Work out the finished part from the listing and answer in its coordinate system (mm). A direction names the side the tool comes from. Coordinates: 2 decimals unless noted, no trailing zeros. Loops run counter-clockwise (first coordinate to the right, second up) from the corner with the lowest first, then second, coordinate; pieces in that order, holes last.
```python
from build123d import *

# Parameters (mm, degrees)
BOSS_EXTRUDE1_DEPTH             = 7.5
F_2_CLEARANCE_HOLE1_D           = 2.2606
F_3_CLEARANCE_HOLE1_D           = 2.6416
F_3_CLEARANCE_HOLE1_CSINK_D     = 4.318
F_3_CLEARANCE_HOLE1_CSINK_ANGLE = 90
FILLET1_R                       = 3


with BuildPart() as part:
    # Sketch3 → Boss-Extrude1 (new body, symmetric)
    with BuildSketch(Plane(origin=(0, 0, 0), x_dir=(1, 0, 0), z_dir=(0, 1, 0))):
        Polygon((0, 0), (0, 20), (3.175, 20), (3.175, 3.175), (15, 3.175), (15, 0), align=None)
    extrude(amount=BOSS_EXTRUDE1_DEPTH, both=True)

    # #2 Clearance Hole1 (through all)
    with Locations(Plane.XY):
        with Locations((10, -3.25), (10, 3.25)):
            Hole(F_2_CLEARANCE_HOLE1_D / 2)

    # #3 Clearance Hole1 (through all)
    with Locations(Plane(origin=(3.175, 0, 0), x_dir=(0, 0, -1), z_dir=(1, 0, 0))):
        with Locations((7.3375, 0), (15.8375, 0)):
            CounterSinkHole(F_3_CLEARANCE_HOLE1_D / 2, F_3_CLEARANCE_HOLE1_CSINK_D / 2, counter_sink_angle=F_3_CLEARANCE_HOLE1_CSINK_ANGLE)

    # Fillet1
    fillet1_edges = [part.edges().sort_by_distance(p)[0] for p in [
        (1.5875, 7.5, -20),
        (1.5875, -7.5, -20),
        (15, -7.5, -1.5875),
        (15, 7.5, -1.5875),
    ]]
    fillet(fillet1_edges, radius=FILLET1_R)


solid = part.part
```
1. A cutting plane is placed at C-C, the plane z = -1.25. Give the vertices of the cut face in (x, y), then the cut area to 3 significant figures.
2. For faces 4 (the flat face through (8, 0, 0)), 5 (the flat face through (9, 0, -3.175)), determine the directions among +Z, -Z, +X, -X, +Y, -Y from which every point of the face is accessible in a straight line to the end or side of a thin tool.
3. Determine the mould class of faces 1 (the cylindrical face through (11.13, -3.2, -1.61)), 2 (the cylindrical face through (1.15, -0.8, -8.39)), 3 (the cylindrical face through (1.61, 6.6, -19.14)) for opening direction Z: released by +Z, released by -Z, zero draft, split by the parting line, or undercut.
4. A cutting plane is placed at A-A, the plane y = 3.25. Give the vertices of the cut face in (x, z) (3 decimals), then the cut area to 3 significant figures.
5. Straight lines are drawn through the part: probe 1 along Z at (x, y) = (0.9, 0); probe 2 along Y at (x, z) = (10, -1.3); probe 3 along Z at (x, y) = (10, -5.5) (3 decimals). For each, find the intervals that lie inside material, in ascending order.
6. A cutting plane is placed at B-B, the plane x = 10. Give the vertices of the cut face in (y, z) (3 decimals), then the cut area to 3 significant figures.
7. A cutting plane is placed at D-D, the plane y = -2.5. Give the vertices of the cut face in (x, z) (3 decimals).
8. Each of these flat-tipped pins is pushed along its axis until it touches: P1, Ø5, axis at y = 6, z = -6.5, coming from the +X side (3 decimals); P2, Ø3.5, axis at x = 11, y = 2.5, coming from the -Z side (3 decimals). Where does it stop, or does it pass through?
Answers below:
1. outline: (0, -7.5) - (12, -7.5) arc R3 ccw to (15, -4.5) - (15, 4.5) arc R3 ccw to (12, 7.5) - (0, 7.5) - close; hole circle Ø2.26 at (10, -3.25); hole circle Ø2.26 at (10, 3.25)
1. area: 213 mm2
2. face 4: +Z, +X, -X, +Y, -Y
2. face 5: -Z, +X, +Y, -Y
3. face 1: zero draft
3. face 2: undercut
3. face 3: released by -Z
4. outline: (0, -20) - (3.175, -20) - (3.175, -3.175) - (8.87, -3.175) - (8.87, 0) - (0, 0) - close; (11.13, -3.175) - (15, -3.175) - (15, 0) - (11.13, 0) - close
4. area: 93.9 mm2
5. probe 1: z = -20 to -17.16, -14.52 to -8.66, -6.02 to 0
5. probe 2: y = -7.5 to -4.38, -2.12 to 2.12, 4.38 to 7.5
5. probe 3: z = -3.175 to 0
6. outline: (-7.5, -3.175) - (-4.38, -3.175) - (-4.38, 0) - (-7.5, 0) - close; (-2.12, -3.175) - (2.12, -3.175) - (2.12, 0) - (-2.12, 0) - close; (4.38, -3.175) - (7.5, -3.175) - (7.5, 0) - (4.38, 0) - close
6. area: 33.3 mm2
7. outline: (0, -20) - (3.175, -20) - (3.175, -3.175) - (9.154, -3.175) - (9.154, 0) - (0, 0) - close; (10.846, -3.175) - (15, -3.175) - (15, 0) - (10.846, 0) - close
8. P1: stops at x = 3.175
8. P2: stops at z = -3.175
